```python
from build123d import *

# Parameters (mm, degrees)
PAD_DEPTH    = 5
PAD001_DEPTH = 60
FILLET_R     = 26
SKETCH002_R  = 2.5
POCKET_DEPTH = 5


with BuildPart() as part:
    # Sketch → Pad (new body)
    with BuildSketch(Plane.XY):
        Polygon((0, 0), (10, 10), (60, 10), (70, 0), align=None)
    extrude(amount=PAD_DEPTH)

    # Sketch001 (on Face6 of Pad) → Pad001 (join)
    with BuildSketch(Plane.XY.offset(5)):
        Polygon((0, 0), (10, 10), (60, 10), (70, 0), (67.172, 0), (59.172, 8), (10.828, 8), (2.828, 0), align=None)
    extrude(amount=PAD001_DEPTH)

    # Fillet
    fillet_edges = [part.edges().sort_by_distance(p)[0] for p in [
        (59.172, 8, 35),
        (10.828, 8, 35),
    ]]
    fillet(fillet_edges, radius=FILLET_R)

    # Sketch002 (on Face1 of Fillet) → Pocket (cut)
    with BuildSketch(Plane.XY.offset(5)):
        with Locations((24, 3)):
            Circle(SKETCH002_R)
        with Locations((46, 3)):
            Circle(SKETCH002_R)
    extrude(amount=-POCKET_DEPTH, mode=Mode.SUBTRACT)


solid = part.part
```
For this review, take the finished solid that the model builds, in its own axes (mm). A direction names the side the tool comes from. Coordinates: 2 decimals unless noted, no trailing zeros. Order: outer loops, then holes, each group sorted by start corner. A loop starts at its lowest first (then second) coordinate and runs counter-clockwise, first axis right, second up. Notation, with made-up numbers: (49.5, 35) - (106.5, 35) arc R24 cw to (106.5, 48) - close; hole circle Ø9 at (62.5, -34.5). An arc over 180 degrees is marked (long way). Answer as a JSON object with one key per item and string values. Group by question number.
1. We need section A-A on x = 24. State the section outline as (y, z) points.
2. For probe 1 along Y at (x, z) = (46, 3); probe 2 along Z at (x, y) = (63.5, 1.5); probe 3 along X at (y, z) = (2.5, 44.5), list the stretches that pass through material, from the lowest coordinate up.
3. We need section D-D on z = 19. State the section outline as (x, y) points, then the cut area to 3 significant figures.
4. We need section B-B on y = 4.5. State the section outline as (x, z) points.
5. Clearance check with flat-ended pins moving along their axes: P1, Ø1.5, axis at x = 29.5, y = 6, coming from the -Z side; P2, Ø5, axis at y = 5.5, z = 49.5, coming from the -X side; P3, Ø1.5, axis at y = 2, z = 24, coming from the +X side; P4, Ø6, axis at x = 24, y = 3, coming from the +Z side. State where each tip first meets the part, or that it passes through.
6. The part is to be moulded in two halves that separate along X. For faces 3 (the flat face through (35, 8, 35)), 4 (the flat face through (5, 5, 32)), 5 (the flat face through (35, 5, 0)), 6 (the cylindrical face through (22, 1.5, 2.5)), say which applies: pulls with the +X half, pulls with the -X half, needs draft (parallel to the pull), parting line crosses it, or undercut.
7. For faces 1 (the flat face through (38, 0, 3)), 2 (the cylindrical face through (58.22, 6.075, 35.42)), list the 3-axis set-ups (+Z, -Z, +X, -X, +Y, -Y) from which the entire face can be reached by the end or side of a thin tool; tool diameter is ignored.
8. We need section C-C on z = 4. State the section outline as (x, y) points, then the cut area to 3 significant figures.
Final values:
{
 "1": {"outline": "(0, 0) - (0.5, 0) - (0.5, 5) - (0, 5) - close; (5.5, 0) - (10, 0) - (10, 65) - (8, 65) - (8, 5) - (5.5, 5) - close"},
 "2": {"probe 1": "0 to 0.5, 5.5 to 10", "probe 2": "0 to 5", "probe 3": "2.5 to 5.61, 64.39 to 67.5"},
 "3": {"outline": "(0, 0) - (2.83, 0) - (3.21, 0.38) arc R26 cw to (21.6, 8) - (48.4, 8) arc R26 cw to (66.79, 0.38) - (67.17, 0) - (70, 0) - (60, 10) - (10, 10) - close", "area": "178 mm²"},
 "4": {"outline": "(4.5, 0) - (22, 0) - (22, 5) - (8.57, 5) - (8.57, 65) - (4.5, 65) - close; (26, 0) - (44, 0) - (44, 5) - (26, 5) - close; (48, 0) - (65.5, 0) - (65.5, 65) - (61.43, 65) - (61.43, 5) - (48, 5) - close"},
 "5": {"P1": "z = 0", "P2": "x = 3", "P3": "x = 68.75", "P4": "z = 5"},
 "6": {"face 3": "undercut", "face 4": "pulls with the -X half", "face 5": "needs draft", "face 6": "undercut"},
 "7": {"face 1": "+Z, -Z, +X, -X, -Y", "face 2": "+Z, -Y"},
 "8": {"outline": "(0, 0) - (70, 0) - (60, 10) - (10, 10) - close; hole circle Ø5 at (24, 3); hole circle Ø5 at (46, 3)", "area": "561 mm²"}
}
